from build123d import *

# Parameters (mm, degrees)
SKETCH1_R           = 2
SKETCH1_R_2         = 1.85
SKETCH1_W           = 8
SKETCH1_H           = 3
BOSS_EXTRUDE1_DEPTH = 1.5


with BuildPart() as part:
    # Sketch1 → Boss-Extrude1 (new body, symmetric)
    with BuildSketch(Plane.XY):
        with BuildLine():
            Line((-27.5, 0), (27.5, 0))
            ThreePointArc((27.5, 0), (36.5, 9), (27.5, 18))
            Line((27.5, 18), (11.1, 18))
            ThreePointArc((11.1, 18), (4.028932188, 20.928932188), (1.1, 28))
            Line((1.1, 28), (1.1, 33))
            ThreePointArc((1.1, 33), (-6.9, 41), (-14.9, 33))
            Line((-14.9, 33), (-14.9, 22))
            ThreePointArc((-14.9, 22), (-17.828932188, 14.928932188), (-24.9, 12))
            Line((-24.9, 12), (-27.5, 12))
            ThreePointArc((-27.5, 12), (-33.5, 6), (-27.5, 0))
        make_face()
        with Locations((-27.5, 6)):
            Circle(SKETCH1_R, mode=Mode.SUBTRACT)
        with Locations((27.5, 9)):
            Circle(SKETCH1_R_2, mode=Mode.SUBTRACT)
        with Locations((-6.9, 33)):
            Circle(SKETCH1_R, mode=Mode.SUBTRACT)
        with Locations((-8.5, 6)):
            Rectangle(SKETCH1_W, SKETCH1_H, mode=Mode.SUBTRACT)
        with Locations((9.5, 6)):
            Rectangle(SKETCH1_W, SKETCH1_H, mode=Mode.SUBTRACT)
    extrude(amount=BOSS_EXTRUDE1_DEPTH, both=True)


solid = part.part
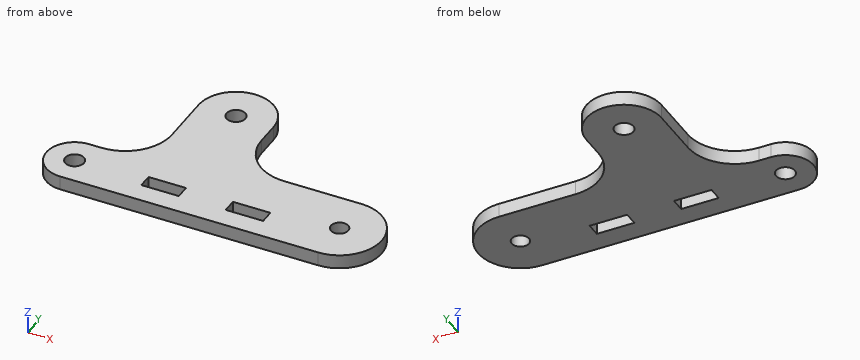
The model under review builds one solid part; all positions refer to its coordinate system, in mm. Round coordinates to 2 decimals unless told otherwise and drop trailing zeros. Order: outer loops, then holes, each group sorted by start corner. A loop starts at its lowest first (then second) coordinate and runs counter-clockwise, first axis right, second up. Notation, with made-up numbers: (-32.5, 78.5) -> (-13.5, 78.5) arc R25 cw to (-13.5, 93.5) -> close; hole circle Ø11 at (-36.5, -30.5). An arc over 180 degrees is marked (long way). Write item = value, one per line. Start each with the question number.
Item 1: Consider section C-C on y = 6. Write out the cut boundary in (x, z).
Item 2: For line 1 along Y through (x, z) = (-5.5, -1.1); line 2 along Y through (x, z) = (-27.5, 0.2); line 3 along Y through (x, z) = (20.5, -1.05), list the stretches that pass through material, from the lowest coordinate up.
Item 3: Consider section A-A on z = 0.95. Write out the cut boundary in (x, y), plus the area to 3 significant figures.
Item 4: Clearance check with flat-ended pins moving along their axes: pin 1 Ø5 at (x, y) = (-6.9, 33) entering from -Z; pin 2 Ø1.5 at (x, z) = (10, -0.5) entering from +Y; pin 3 Ø1 at (x, z) = (8.5, 0) entering from +Y; pin 4 Ø1.5 at (y, z) = (31.5, 0) entering from +X. State where each tip first meets the part, or that it passes through.
Item 5: Consider section B-B on x = -6.9. Write out the cut boundary in (y, z), plus the area to 3 significant figures.
Item 6: Consider section D-D on x = 8. Write out the cut boundary in (y, z).
Conclusion:
q1.outline = (-33.5, -1.5) -> (-29.5, -1.5) -> (-29.5, 1.5) -> (-33.5, 1.5) -> close; (-25.5, -1.5) -> (-12.5, -1.5) -> (-12.5, 1.5) -> (-25.5, 1.5) -> close; (-4.5, -1.5) -> (5.5, -1.5) -> (5.5, 1.5) -> (-4.5, 1.5) -> close; (13.5, -1.5) -> (35.99, -1.5) -> (35.99, 1.5) -> (13.5, 1.5) -> close
q2.line_1 = 0 to 4.5, 7.5 to 31.57, 34.43 to 40.88
q2.line_2 = 0 to 4, 8 to 12
q2.line_3 = 0 to 18
q3.outline = (-27.5, 0) -> (27.5, 0) arc R9 ccw to (27.5, 18) -> (11.1, 18) arc R10 cw to (1.1, 28) -> (1.1, 33) arc R8 ccw to (-14.9, 33) -> (-14.9, 22) arc R10 cw to (-24.9, 12) -> (-27.5, 12) arc R6 ccw to start; hole circle Ø4 at (-27.5, 6); hole (-12.5, 4.5) -> (-4.5, 4.5) -> (-4.5, 7.5) -> (-12.5, 7.5) -> close; hole circle Ø4 at (-6.9, 33); hole (5.5, 4.5) -> (13.5, 4.5) -> (13.5, 7.5) -> (5.5, 7.5) -> close; hole circle Ø3.7 at (27.5, 9)
q3.area = 1,400 mm2
q4.pin_1 = -1.5
q4.pin_2 = 18.17
q4.pin_3 = 18.49
q4.pin_4 = 1.1
q5.outline = (0, -1.5) -> (4.5, -1.5) -> (4.5, 1.5) -> (0, 1.5) -> close; (7.5, -1.5) -> (31, -1.5) -> (31, 1.5) -> (7.5, 1.5) -> close; (35, -1.5) -> (41, -1.5) -> (41, 1.5) -> (35, 1.5) -> close
q5.area = 102 mm2
q6.outline = (0, -1.5) -> (4.5, -1.5) -> (4.5, 1.5) -> (0, 1.5) -> close; (7.5, -1.5) -> (18.49, -1.5) -> (18.49, 1.5) -> (7.5, 1.5) -> close
